from build123d import *

# Parameters (mm, degrees)
SKETCH1_W           = 36
SKETCH1_H           = 49
BOSS_EXTRUDE2_DEPTH = 90
SHELL3_T            = -4
FILLET1_R           = 2
FILLET2_R           = 2
FILLET3_R           = 2
FILLET4_R           = 2
FILLET5_R           = 2
SKETCH7_W           = 1.5
SKETCH7_H           = 5
SKETCH7_W_2         = 1.499999997
SKETCH7_W_3         = 5
SKETCH7_H_2         = 2
BOSS_EXTRUDE3_DEPTH = 7
SKETCH8_W           = 2
SKETCH8_H           = 5
BOSS_EXTRUDE4_DEPTH = 5
SKETCH9_W           = 2
SKETCH9_H           = 5
BOSS_EXTRUDE5_DEPTH = 5
SKETCH10_W          = 2
SKETCH10_H          = 5
BOSS_EXTRUDE6_DEPTH = 5
FILLET7_R           = 2
FILLET8_R           = 2
FILLET9_R           = 2
FILLET10_R          = 2


with BuildPart() as part:
    # Sketch1 → Boss-Extrude2 (new body)
    with BuildSketch(Plane(origin=(0, 0, 0), x_dir=(1, 0, 0), z_dir=(0, 1, 0))):
        with Locations((3.176470588, -4.072192513)):
            Rectangle(SKETCH1_W, SKETCH1_H)
    extrude(amount=BOSS_EXTRUDE2_DEPTH)

    # Shell3
    shell3_openings = [part.faces().sort_by_distance(p)[0] for p in [
        (3.176470588, 90, 4.072192513),
    ]]
    offset(amount=SHELL3_T, openings=shell3_openings, kind=Kind.INTERSECTION)

    # Fillet1
    fillet1_edges = [part.edges().sort_by_distance(p)[0] for p in [
        (-14.823529412, 45, -20.427807487),
    ]]
    fillet(fillet1_edges, radius=FILLET1_R)

    # Fillet2
    fillet2_edges = [part.edges().sort_by_distance(p)[0] for p in [
        (21.176470588, 45, -20.427807487),
    ]]
    fillet(fillet2_edges, radius=FILLET2_R)

    # Fillet3
    fillet3_edges = [part.edges().sort_by_distance(p)[0] for p in [
        (21.176470588, 45, 28.572192513),
    ]]
    fillet(fillet3_edges, radius=FILLET3_R)

    # Fillet4
    fillet4_edges = [part.edges().sort_by_distance(p)[0] for p in [
        (-14.823529412, 45, 28.572192513),
    ]]
    fillet(fillet4_edges, radius=FILLET4_R)

    # Fillet5
    fillet5_edges = [part.edges().sort_by_distance(p)[0] for p in [
        (-14.823529412, 0, 4.072192513),
        (3.176470588, 0, -20.427807487),
        (21.176470588, 0, 4.072192513),
        (3.176470588, 0, 28.572192513),
    ]]
    fillet(fillet5_edges, radius=FILLET5_R)

    # Sketch7 → Boss-Extrude3 (add)
    with BuildSketch(Plane(origin=(21.176470588, 0, 0), x_dir=(0, 0, -1), z_dir=(1, 0, 0))):
        with Locations((-23.322192513, 29.805726248)):
            Rectangle(SKETCH7_W, SKETCH7_H)
        with Locations((14.177807489, 29.805726248)):
            Rectangle(SKETCH7_W_2, SKETCH7_H)
        with Locations((-4.572192513, 11.305726248)):
            Rectangle(SKETCH7_W_3, SKETCH7_H_2)
    extrude(amount=BOSS_EXTRUDE3_DEPTH)

    # Sketch8 → Boss-Extrude4 (add)
    with BuildSketch(Plane(origin=(0, 0, 22.572192513), x_dir=(-1, 0, 0), z_dir=(0, 0, -1))):
        with Locations((-27.176470588, 29.805726248)):
            Rectangle(SKETCH8_W, SKETCH8_H)
    extrude(amount=BOSS_EXTRUDE4_DEPTH)

    # Sketch9 → Boss-Extrude5 (add)
    with BuildSketch(Plane.XY.offset(-13.42780749)):
        with Locations((27.176470588, 29.805726248)):
            Rectangle(SKETCH9_W, SKETCH9_H)
    extrude(amount=BOSS_EXTRUDE5_DEPTH)

    # Sketch10 → Boss-Extrude6 (add)
    with BuildSketch(Plane(origin=(0, 12.305726248, 0), x_dir=(1, 0, 0), z_dir=(0, 1, 0))):
        with Locations((27.176470588, -4.572192513)):
            Rectangle(SKETCH10_W, SKETCH10_H)
    extrude(amount=BOSS_EXTRUDE6_DEPTH)

    # Fillet7
    fillet7_edges = [part.edges().sort_by_distance(p)[0] for p in [
        (17.176470588, 90, 4.072192513),
    ]]
    fillet(fillet7_edges, radius=FILLET7_R)

    # Fillet8
    fillet8_edges = [part.edges().sort_by_distance(p)[0] for p in [
        (3.176470588, 90, -16.427807487),
    ]]
    fillet(fillet8_edges, radius=FILLET8_R)

    # Fillet9
    fillet9_edges = [part.edges().sort_by_distance(p)[0] for p in [
        (-10.823529412, 90, 4.072192513),
    ]]
    fillet(fillet9_edges, radius=FILLET9_R)

    # Fillet10
    fillet10_edges = [part.edges().sort_by_distance(p)[0] for p in [
        (3.176470588, 90, 24.572192513),
    ]]
    fillet(fillet10_edges, radius=FILLET10_R)


solid = part.part
Read the model definition and answer for the solid it produces. Units are mm, in the model's axes. A direction names the side the tool comes from. Give positions to 0.01 mm unless a question says otherwise; leave off trailing zeros. Loops run counter-clockwise (first coordinate to the right, second up) from the corner with the lowest first, then second, coordinate; pieces in that order, holes last. Notation, with made-up numbers: (-11.75, 23) -> (38.25, 23) arc R23 cw to (38.25, 42) -> close; hole circle Ø7 at (-34, 63.5). An arc over 180 degrees is marked (long way). Answer as CSV lines item,"result".
Item 1: Find section A-A on y = 15. Give the vertices of the cut face in (x, z), plus the area to 3 significant figures.
Returned:
outline,"(-14.82, -18.43) arc R2 ccw to (-12.82, -20.43) -> (19.18, -20.43) arc R2 ccw to (21.18, -18.43) -> (21.18, 26.57) arc R2 ccw to (19.18, 28.57) -> (-12.82, 28.57) arc R2 ccw to (-14.82, 26.57) -> close; (26.18, 2.07) -> (28.18, 2.07) -> (28.18, 7.07) -> (26.18, 7.07) -> close; hole (-10.82, -16.43) -> (17.18, -16.43) -> (17.18, 24.57) -> (-10.82, 24.57) -> close"
area,"623 mm²"
Item 2: For faces 1 (the face through (25, 12, 2.072)), 2 (the face through (26.176, 30, -11)), 3 (the face through (3, 45, 24.572)), 4 (the face through (27, 17.306, 5)), determine the directions among +Z, -Z, +X, -X, +Y, -Y from which every point of the face is accessible in a straight line to the end or side of a thin tool.
Returned:
face 1,"-Z, +X, +Y, -Y"
face 2,"+Y, -Y"
face 3,"+Y"
face 4,"+Z, -Z, +X, +Y"
Item 3: Find section B-B on x = 1. Give the vertices of the cut face in (y, z).
Returned:
outline,"(0, -18.43) arc R2 ccw to (2, -20.43) -> (90, -20.43) -> (90, -18.43) arc R2 ccw to (88, -16.43) -> (4, -16.43) -> (4, 24.57) -> (88, 24.57) arc R2 ccw to (90, 26.57) -> (90, 28.57) -> (2, 28.57) arc R2 ccw to (0, 26.57) -> close"
Item 4: Determine the mould class of faces 5 (the face through (-14.25, 46.62, -19.83)), 6 (the face through (17.78, 89.43, 4.39)), 7 (the face through (20.575, 46.616, -19.857)), 8 (the face through (3, 45, 28.572)) for opening direction X: +X half, -X half, draft (parallel to the pull), parting line (faces both ways), or undercut.
Returned:
face 5,"-X half"
face 6,"undercut"
face 7,"+X half"
face 8,"draft"
Item 5: Each of these flat-tipped pins is pushed along its axis until it touches: pin 1 (20.5 mm diameter, centred on y = 52, z = -1.5, fed in from +X); pin 2 (6 mm diameter, centred on x = -9.5, z = -12, fed in from +Y); pin 3 (3 mm diameter, centred on x = 26.5, z = 22, fed in from +Y). Where does it stop, or does it pass through?
Returned:
pin 1,"stops at x = 21.18"
pin 2,"stops at y = 89.97"
pin 3,"stops at y = 32.31"
Item 6: Find section C-C on y = 61. Give the vertices of the cut face in (x, z), plus the area to 3 significant figures.
Returned:
outline,"(-14.82, -18.43) arc R2 ccw to (-12.82, -20.43) -> (19.18, -20.43) arc R2 ccw to (21.18, -18.43) -> (21.18, 26.57) arc R2 ccw to (19.18, 28.57) -> (-12.82, 28.57) arc R2 ccw to (-14.82, 26.57) -> close; hole (-10.82, -16.43) -> (17.18, -16.43) -> (17.18, 24.57) -> (-10.82, 24.57) -> close"
area,"613 mm²"
Item 7: Consider line 1 (Z direction, x = -8, y = 11); line 2 (X direction, y = 65, z = -10); line 3 (Z direction, x = -13, y = 78). Determine where each line is inside the solid, lowest interval first. Write a range as [from, to].
Returned:
line 1,"z = [-20.43, -16.43], [24.57, 28.57]"
line 2,"x = [-14.82, -10.82], [17.18, 21.18]"
line 3,"z = [-20.42, 28.56]"
Item 8: Find section D-D on z = -7.5. Give the vertices of the cut face in (x, y).
Returned:
outline,"(-14.82, 2) arc R2 ccw to (-12.82, 0) -> (19.18, 0) arc R2 ccw to (21.18, 2) -> (21.18, 90) -> (19.18, 90) arc R2 ccw to (17.18, 88) -> (17.18, 4) -> (-10.82, 4) -> (-10.82, 88) arc R2 ccw to (-12.82, 90) -> (-14.82, 90) -> close"
